Read the model definition and answer for the solid it produces. Units are mm, in the model's axes. A direction names the side the tool comes from. Round coordinates to 2 decimals unless told otherwise and drop trailing zeros. Order: outer loops, then holes, each group sorted by start corner. A loop starts at its lowest first (then second) coordinate and runs counter-clockwise, first axis right, second up. Notation, with made-up numbers: (77.25, 3) -> (130.25, 3) arc R4 cw to (130.25, 7) -> close; hole circle Ø3 at (58, 72.5). An arc over 180 degrees is marked (long way). Answer as a JSON object with one key per item and string values. Group by question number.
Item 1: Consider probe 1 along Y at (x, z) = (0, 45); probe 2 along X at (y, z) = (0, 14); probe 3 along X at (y, z) = (-28, 30). Determine where each line is inside the solid, lowest interval first. Write a range as from..to.
Item 2: Section A-A, the plane x = 13 is taken. Write down the section's boundary in (y, z).
Item 3: For faces 4 (the cylindrical face through (-8, -29, 35)), 5 (the cylindrical face through (29.77, 1.46, 35.49)), 6 (the flat face through (4, 19, 35)), determine the directions among +Z, -Z, +X, -X, +Y, -Y from which every point of the face is accessible in a straight line to the end or side of a thin tool.
Item 4: Section B-B, the plane y = 5 is taken. Write down the section's boundary in (x, z).
Item 5: The mould has two halves that part along Y. Classify faces 1 (the cylindrical face through (8, 29, 35)), 2 (the cylindrical face through (-21.005, 21.15, 35.49)), 3 (the cylindrical face through (1.69, -29.82, 35.49)): pulls with the +Y half, pulls with the -Y half, needs draft (parallel to the pull), parting line crosses it, or undercut.
Item 6: Given P1, Ø10, axis at x = -8, z = 24, coming from the -Y side; P2, Ø3.5, axis at y = 18, z = 26.5, coming from the -X side; P3, Ø6, axis at y = 23.5, z = 41.5, coming from the +X side, each flat-ended and moving along its own axis, determine where each tip first touches the part or whether it passes through.
from build123d import *

# Parameters (mm, degrees)
SKETCH1_R           = 32
BOSS_EXTRUDE1_DEPTH = 70
CUT_EXTRUDE1_DEPTH  = 70
CIRPATTERN1_COUNT   = 30
CUT_EXTRUDE2_DEPTH  = 70


with BuildPart() as part:
    # Sketch1 → Boss-Extrude1 (new body)
    with BuildSketch(Plane.XY):
        Circle(SKETCH1_R)
    extrude(amount=BOSS_EXTRUDE1_DEPTH)

    # Sketch3 → Cut-Extrude1 (cut)
    with BuildSketch(Plane.XY.offset(70)):
        with BuildLine():
            Line((3.082235405, 32), (-3.082235405, 32))
            ThreePointArc((-3.082235405, 32), (-1.716298742, 29.871791027), (-0.838993939, 27.5))
            Line((-0.838993939, 27.5), (0.838993939, 27.5))
            ThreePointArc((0.838993939, 27.5), (1.716298742, 29.871791027), (3.082235405, 32))
        make_face()
    cut_extrude1 = extrude(amount=-CUT_EXTRUDE1_DEPTH, mode=Mode.SUBTRACT)

    # CirPattern1: Cut-Extrude1 ×30 about axis
    cirpattern1_axis = Axis((0, 0, 0), (0, 0, 1))
    for i in range(1, CIRPATTERN1_COUNT):
        add(cut_extrude1.rotate(cirpattern1_axis, i * 360 / CIRPATTERN1_COUNT), mode=Mode.SUBTRACT)

    # Sketch4 → Cut-Extrude2 (cut)
    with BuildSketch(Plane.XY.offset(70)):
        with BuildLine():
            Line((-4, 17.036725037), (-4, 20.036725037))
            Line((-4, 20.036725037), (4, 20.036725037))
            Line((4, 20.036725037), (4, 17.036725037))
            ThreePointArc((4, 17.036725037), (0, -17.5), (-4, 17.036725037))
        make_face()
    extrude(amount=-CUT_EXTRUDE2_DEPTH, mode=Mode.SUBTRACT)


solid = part.part
Values found:
{
 "1": {"probe 1": "-27.5..-17.5, 20.04..27.5", "probe 2": "-32..-17.5, 17.5..32", "probe 3": "-10.58..-7.27, -4.83..-0.98, 0.98..4.83, 7.27..10.58"},
 "2": {"outline": "(-25.95, 0) -> (-11.72, 0) -> (-11.72, 70) -> (-25.95, 70) -> close; (11.72, 0) -> (25.95, 0) -> (25.95, 70) -> (11.72, 70) -> close"},
 "3": {"face 4": "+Z, -Z, -Y", "face 5": "+Z, -Z, +X", "face 6": "+Z, -Z"},
 "4": {"outline": "(-29.79, 0) -> (-16.77, 0) -> (-16.77, 70) -> (-29.79, 70) -> close; (16.77, 0) -> (29.79, 0) -> (29.79, 70) -> (16.77, 70) -> close"},
 "5": {"face 1": "pulls with the +Y half", "face 2": "undercut", "face 3": "pulls with the -Y half"},
 "6": {"P1": "y = -31.86", "P2": "x = -26.11", "P3": "x = 21.69"}
}
